```python
from build123d import *

# Parameters (mm, degrees)
SKETCH1_W           = 86.36
SKETCH1_H           = 68.58
BOSS_EXTRUDE1_DEPTH = 3.175
FILLET1_R           = 2.54
SKETCH2_R           = 1.6129
CUT_EXTRUDE1_DEPTH  = 4.175
SKETCH3_W           = 44.145937315
SKETCH3_H           = 4.712813079
SKETCH3_W_2         = 34.939039867
SKETCH3_H_2         = 4.658410012
CUT_EXTRUDE2_DEPTH  = 4.175


with BuildPart() as part:
    # Sketch1 → Boss-Extrude1 (new body)
    with BuildSketch(Plane(origin=(0, 0, 0), x_dir=(1, 0, 0), z_dir=(0, 1, 0))):
        with Locations((43.18, -34.29)):
            Rectangle(SKETCH1_W, SKETCH1_H)
    extrude(amount=BOSS_EXTRUDE1_DEPTH)

    # Fillet1
    fillet1_edges = [part.edges().sort_by_distance(p)[0] for p in [
        (0, 1.5875, 0),
        (86.36, 1.5875, 0),
        (86.36, 1.5875, 68.58),
        (0, 1.5875, 68.58),
    ]]
    fillet(fillet1_edges, radius=FILLET1_R)

    # Sketch2 → Cut-Extrude1 (cut, through all)
    with BuildSketch(Plane(origin=(0, 3.175, 0), x_dir=(-1, 0, 0), z_dir=(0, 1, 0))):
        with Locations(Location((-4.054045308, 3.152222292, 0), (0, 0, 90))):  # turned: the seam where the file's is
            Circle(SKETCH2_R)
        with Locations(Location((-83.076051224, 3.283948776, 0), (0, 0, 90))):  # turned: the seam where the file's is
            Circle(SKETCH2_R)
        with Locations(Location((-82.305954692, 65.427777708, 0), (0, 0, 90))):  # turned: the seam where the file's is
            Circle(SKETCH2_R)
        with Locations(Location((-4.054045308, 65.427777708, 0), (0, 0, 90))):  # turned: the seam where the file's is
            Circle(SKETCH2_R)
    extrude(amount=-CUT_EXTRUDE1_DEPTH, mode=Mode.SUBTRACT)

    # Sketch3 → Cut-Extrude2 (cut, through all)
    with BuildSketch(Plane(origin=(0, 3.175, 0), x_dir=(1, 0, 0), z_dir=(0, 1, 0))):
        with Locations((55.366118113, -8.634348767)):
            Rectangle(SKETCH3_W, SKETCH3_H)
        with Locations((60.97547331, -57.248737221)):
            Rectangle(SKETCH3_W_2, SKETCH3_H_2)
    extrude(amount=-CUT_EXTRUDE2_DEPTH, mode=Mode.SUBTRACT)


solid = part.part
```
Model file for the job. Use its own axes, mm. A direction names the side the tool comes from. Coordinates: 2 decimals unless noted, no trailing zeros. Order: outer loops, then holes, each group sorted by start corner. A loop starts at its lowest first (then second) coordinate and runs counter-clockwise, first axis right, second up. Notation, with made-up numbers: (-12.75, 30) -> (43.25, 30) arc R26 ccw to (43.25, 56) -> close; hole circle Ø4 at (-19.5, 43). An arc over 180 degrees is marked (long way). Answer as a JSON object with one key per item and string values. Group by question number.
1) Drill centre lines: L1, parallel to Z at x = 68, y = 1.05; L2, parallel to X at y = 2.3, z = 65.5; L3, parallel to Z at x = 41, y = 0.55. Where is each one in solid material? Low to high.
2) Cut at A-A, the plane z = 56. Write the cut outline in (x, y) (3 decimals).
3) Cut at B-B, the plane x = 37. Write the cut outline in (y, z) (3 decimals), then the cut area to 3 significant figures.
4) Which spindle directions (+Z, -Z, +X, -X, +Y, -Y) get a long thin tool onto all of the face, cutting with end or side? Do faces 1 (the face through (86.36, 2, 35)), 2 (the face through (55, 2, 10.991)). Say none if no direction does.
5) Cut at C-C, the plane x = 51.5. Write the cut outline in (y, z) (3 decimals).
6) Cut at D-D, the plane y = 1.75. Write the cut outline in (x, z) (3 decimals).
7) Pull direction X, two halves, no side cores. Call faces 3 (the face through (85.596, 1.61, 67.856)), 4 (the face through (43, 2, 68.58)), 5 (the face through (61, 2, 59.578)): +X half, -X half, draft (parallel to the pull), parting line (faces both ways), or undercut.
Check values:
{
 "1": {"L1": "z = 0 to 6.28, 10.99 to 54.92, 59.58 to 68.58", "L2": "x = 0 to 2.44, 5.67 to 80.69, 83.92 to 86.36", "L3": "z = 0 to 6.28, 10.99 to 68.58"},
 "2": {"outline": "(0, 0) -> (43.506, 0) -> (43.506, 3.175) -> (0, 3.175) -> close; (78.445, 0) -> (86.36, 0) -> (86.36, 3.175) -> (78.445, 3.175) -> close"},
 "3": {"outline": "(0, 0) -> (3.175, 0) -> (3.175, 6.278) -> (0, 6.278) -> close; (0, 10.991) -> (3.175, 10.991) -> (3.175, 68.58) -> (0, 68.58) -> close", "area": "203 mm²"},
 "4": {"face 1": "+Z, -Z, +X, +Y, -Y", "face 2": "+Y, -Y"},
 "5": {"outline": "(0, 0) -> (3.175, 0) -> (3.175, 6.278) -> (0, 6.278) -> close; (0, 10.991) -> (3.175, 10.991) -> (3.175, 54.92) -> (0, 54.92) -> close; (0, 59.578) -> (3.175, 59.578) -> (3.175, 68.58) -> (0, 68.58) -> close"},
 "6": {"outline": "(0, 2.54) arc R2.54 ccw to (2.54, 0) -> (83.82, 0) arc R2.54 ccw to (86.36, 2.54) -> (86.36, 66.04) arc R2.54 ccw to (83.82, 68.58) -> (2.54, 68.58) arc R2.54 ccw to (0, 66.04) -> close; hole circle Ø3.226 at (4.054, 3.152); hole circle Ø3.226 at (4.054, 65.428); hole (33.293, 6.278) -> (77.439, 6.278) -> (77.439, 10.991) -> (33.293, 10.991) -> close; hole (43.506, 54.92) -> (78.445, 54.92) -> (78.445, 59.578) -> (43.506, 59.578) -> close; hole circle Ø3.226 at (82.306, 65.428); hole circle Ø3.226 at (83.076, 3.284)"},
 "7": {"face 3": "+X half", "face 4": "draft", "face 5": "undercut"}
}
